```python
from build123d import *

# Parameters (mm, degrees)
SKETCH1_R               = 3.175
BOSS_EXTRUDE1_DEPTH     = 31.75
SKETCH2_R               = 6.35
BOSS_EXTRUDE2_DEPTH     = 2.54
CUT_EXTRUDE1_DEPTH      = 33.995567884
CUT_EXTRUDE1_DEPTH_BACK = 33.995567884
SKETCH3_R               = 1.75
FILLET2_R               = 0.635


with BuildPart() as part:
    # Sketch1 → Boss-Extrude1 (new body)
    with BuildSketch(Plane.XY):
        Circle(SKETCH1_R)
    extrude(amount=BOSS_EXTRUDE1_DEPTH)

    # Sketch2 → Boss-Extrude2 (add)
    with BuildSketch(Plane(origin=(0, 0, 0), x_dir=(-1, 0, 0), z_dir=(0, 0, -1))):
        Circle(SKETCH2_R)
    extrude(amount=BOSS_EXTRUDE2_DEPTH)

    # Sketch3 → Cut-Extrude1 (cut, two sides: drawn at the far end of the back side and taken through both)
    with BuildSketch(Plane(origin=(0, 0, 0), x_dir=(0, 0, -1), z_dir=(1, 0, 0)).offset(-CUT_EXTRUDE1_DEPTH_BACK)):
        with Locations(Location((-27.94, 0, 0), (0, 0, 180.000000003))):
            Circle(SKETCH3_R)
    extrude(amount=CUT_EXTRUDE1_DEPTH + CUT_EXTRUDE1_DEPTH_BACK, mode=Mode.SUBTRACT)

    # Fillet2
    fillet2_edges = [part.edges().sort_by_distance(p)[0] for p in [
        (-3.175, 0, 31.75),
        (6.35, 0, 0),
        (6.35, 0, -2.54),
    ]]
    fillet(fillet2_edges, radius=FILLET2_R)


solid = part.part
```
Could you check a few things on this model? Use its own coordinates, in mm. A direction names the side the tool comes from. Give positions to 0.01 mm unless a question says otherwise; leave off trailing zeros. Loops run counter-clockwise (first coordinate to the right, second up) from the corner with the lowest first, then second, coordinate; pieces in that order, holes last. Notation, with made-up numbers: (-9.5, 67) - (44.5, 67) arc R21 ccw to (44.5, 84) - close; hole circle Ø2 at (-20, 29.25). An arc over 180 degrees is marked (long way). Use one line per item in the form item = value.
1. On a 3-axis mill with a long thin cutter (end or side, diameter ignored), from which of +Z, -Z, +X, -X, +Y, -Y can I reach the whole of each face in a straight line? I mean faces 1 (the face through (0, 0, 31.75)), 2 (the face through (-2.5, -2.5, 0)). Say none if no direction works.
Response values:
face_1 = +Z, +X, -X, +Y, -Y
face_2 = +Z
2. I need wall thicknesses on probe 1 along Z at (x, y) = (0.5, 0); probe 2 along Z at (x, y) = (3, 2.75); probe 3 along Y at (x, z) = (-0.5, 29.5). Which ranges of each line are inside material? Lowest first, please.
Response values:
probe_1 = -2.54 to 26.19, 29.69 to 31.75
probe_2 = -2.54 to 0
probe_3 = -3.14 to -0.79, 0.79 to 3.14
3. I'm going to push flat-ended pins straight in: pin 1 Ø1 at (y, z) = (3, 16.5) entering from +X; pin 2 Ø6 at (y, z) = (-0.5, 14.5) entering from -X (3 decimals); pin 3 Ø3 at (y, z) = (0, 27.94) entering from +X; pin 4 Ø2 at (y, z) = (-3, 25) entering from +X. Where does each tip first touch, or does it pass through?
Response values:
pin_1 = 1.96
pin_2 = -3.175
pin_3 = through
pin_4 = 2.47
4. Thinking about a two-plate mould opening in Z: for faces 3 (the face through (0, 0, -2.54)), 4 (the face through (-0.04, -1.18, 26.65)), 5 (the face through (1.38, -6.2, -1.26)), which applies, released by +Z, released by -Z, zero draft, split by the parting line, or undercut?
Response values:
face_3 = released by -Z
face_4 = undercut
face_5 = zero draft
5. I want a section at A-A (x = 0). Please give me the cut outline in (y, z) (3 decimals).
Response values:
outline = (-6.35, -1.905) arc R0.635 ccw to (-5.715, -2.54) - (5.715, -2.54) arc R0.635 ccw to (6.35, -1.905) - (6.35, -0.635) arc R0.635 ccw to (5.715, 0) - (3.175, 0) - (3.175, 31.115) arc R0.635 ccw to (2.54, 31.75) - (-2.54, 31.75) arc R0.635 ccw to (-3.175, 31.115) - (-3.175, 0) - (-5.715, 0) arc R0.635 ccw to (-6.35, -0.635) - close; hole circle Ø3.5 at (0, 27.94)
6. I want a section at C-C (z = 18). Please give me the cut outline in (x, y) (3 decimals).
Response values:
outline = circle Ø6.35 at (0, 0)
7. I want a section at D-D (z = 27.94). Please give me the cut outline in (x, y) (3 decimals), and give its area (3 significant figures).
Response values:
outline = (-2.649, -1.75) arc R3.175 ccw to (2.649, -1.75) - close; (-2.649, 1.75) - (2.649, 1.75) arc R3.175 ccw to start
area = 10.6 mm²
8. I want a section at B-B (y = 0). Please give me the cut outline in (x, z) (3 decimals).
Response values:
outline = (-6.35, -1.905) arc R0.635 ccw to (-5.715, -2.54) - (5.715, -2.54) arc R0.635 ccw to (6.35, -1.905) - (6.35, -0.635) arc R0.635 ccw to (5.715, 0) - (3.175, 0) - (3.175, 26.19) - (-3.175, 26.19) - (-3.175, 0) - (-5.715, 0) arc R0.635 ccw to (-6.35, -0.635) - close; (-3.175, 29.69) - (3.175, 29.69) - (3.175, 31.115) arc R0.635 ccw to (2.54, 31.75) - (-2.54, 31.75) arc R0.635 ccw to (-3.175, 31.115) - close
